Check sheet for the modelled part. Datum: model origin and axes. Units: mm. Give positions to 0.01 mm unless a question says otherwise; leave off trailing zeros. Order: outer loops, then holes, each group sorted by start corner. A loop starts at its lowest first (then second) coordinate and runs counter-clockwise, first axis right, second up.
Autodesk Inventor part; units mm, degrees
ref_plane "YZ Plane" through (0, 0, 0) normal (1, 0, 0) x (0, 1, 0)
ref_plane "XZ Plane" through (0, 0, 0) normal (0, 1, 0) x (-1, 0, 0)
ref_plane "XY Plane" through (0, 0, 0) normal (0, 0, 1) x (1, 0, 0)
sketch "main" plane through (0, 0, 0) normal (0, 0, 1) x (1, 0, 0)
  circle A0 centre (2.6045, 11.9092) radius 2.1844
  circle A1 centre (-3.5552, 26.8777) radius 2.0955
  arc A2 (-0.6729, 30.669) -> (-7.4873, 29.5648) centre (-3.5552, 26.8777) ccw
  circle A3 centre (19.8371, 7.1) radius 2.0955
  arc A4 (24.7659, 3.0962) -> (23.6801, 12.155) centre (19.8371, 7.1) ccw
  circle A5 centre (-16.2552, -5.1047) radius 2.1844
  circle A6 centre (-0.7959, -18.3) radius 2.0955
  arc A7 (-0.0936, -24.6111) -> (4.1329, -22.3038) centre (-0.7959, -18.3) ccw
  circle A8 centre (-25.6851, -13.6116) radius 2.1844
  line L0 (-34.4127, -28.4296) -> (-0.0936, -24.6111)
  circle A9 centre (-35.1149, -22.1186) radius 2.1844
  arc A10 (-40.3577, -18.5358) -> (-34.4127, -28.4296) centre (-35.1149, -22.1186) ccw
  line L1 (-7.4873, 29.5648) -> (-40.3577, -18.5358)
  line L2 (24.7659, 3.0962) -> (4.1329, -22.3038)
  line L3 (-0.6729, 30.669) -> (23.6801, 12.155)
  point P0 (-5.4325, -4.0149)
  point P1 (-6.8254, 3.4022)
  dimension "d2" = 4.191
  dimension "d3" = 12.7
  dimension "d5" = 12.7
  dimension "d6" = 12.7
  dimension "d8" = 4.191
  dimension "d9" = 9.525
  dimension "d10" = 4.191
  dimension "d13" = 4.3688
sketch "Sketch1" plane through (0, 0, 0) normal (0, 0, 1) x (1, 0, 0)
  circle A0 centre (2.6045, 11.9092) radius 2.1844
  circle A1 centre (-3.5552, 26.8777) radius 2.0955
  arc A2 (-0.6729, 30.669) -> (-7.4873, 29.5648) centre (-3.5552, 26.8777) ccw
  circle A3 centre (19.8371, 7.1) radius 2.0955
  arc A4 (24.7659, 3.0962) -> (23.6801, 12.155) centre (19.8371, 7.1) ccw
  circle A5 centre (-16.2552, -5.1047) radius 2.1844
  circle A6 centre (-0.7959, -18.3) radius 2.0955
  arc A7 (-0.0936, -24.6111) -> (4.1329, -22.3038) centre (-0.7959, -18.3) ccw
  circle A8 centre (-25.6851, -13.6116) radius 2.1844
  line L0 (-34.4127, -28.4296) -> (-0.0936, -24.6111)
  circle A9 centre (-35.1149, -22.1186) radius 2.1844
  arc A10 (-40.3577, -18.5358) -> (-34.4127, -28.4296) centre (-35.1149, -22.1186) ccw
  line L1 (-7.4873, 29.5648) -> (-40.3577, -18.5358)
  line L2 (24.7659, 3.0962) -> (4.1329, -22.3038)
  line L3 (-0.6729, 30.669) -> (23.6801, 12.155)
  point P0 (0, 0)
extrude "Extrusion1" add sketch "Sketch1" along normal blind 1.5875
properties part number "Gearbox" material "Acetal Resin, White"
(1) Release check for a two-part mould opening along Y. For faces 1 (the face through (-8, -5, 0)), 2 (the face through (-23.692, 5.851, 0.783)), 3 (the face through (-36.85, -20.79, 0.78)), 4 (the face through (-40.505, -25.476, 0.783)) record: released by +Y, released by -Y, zero draft, split by the parting line, or undercut.
Response values:
face 1: zero draft
face 2: released by +Y
face 3: undercut
face 4: split by the parting line
(2) Cross-section at C-C on x = -9.5. Enter the section's corners in (y, z), then the cut area to 3 significant figures.
Response values:
outline: (-25.66, 0) - (26.62, 0) - (26.62, 1.59) - (-25.66, 1.59) - close
area: 83.0 mm2
(3) Cross-section at D-D on y = 21.5. Enter the section's corners in (x, z).
Response values:
outline: (-13, 0) - (11.39, 0) - (11.39, 1.59) - (-13, 1.59) - close
(4) Cross-section at B-B on z = 0.9. Enter the section's corners in (x, y) (1 decimal), then the cut area to 3 significant figures.
Response values:
outline: (-40.4, -18.5) arc R6.3 ccw to (-34.4, -28.4) - (-0.1, -24.6) arc R6.4 ccw to (4.1, -22.3) - (24.8, 3.1) arc R6.3 ccw to (23.7, 12.2) - (-0.7, 30.7) arc R4.8 ccw to (-7.5, 29.6) - close; hole circle Ø4.4 at (-35.1, -22.1); hole circle Ø4.4 at (-25.7, -13.6); hole circle Ø4.4 at (-16.3, -5.1); hole circle Ø4.2 at (-3.6, 26.9); hole circle Ø4.2 at (-0.8, -18.3); hole circle Ø4.4 at (2.6, 11.9); hole circle Ø4.2 at (19.8, 7.1)
area: 2,210 mm2
(5) Cross-section at A-A on y = 13. Enter the section's corners in (x, z), then the cut area to 3 significant figures.
Response values:
outline: (-18.81, 0) - (0.71, 0) - (0.71, 1.59) - (-18.81, 1.59) - close; (4.5, 0) - (22.57, 0) - (22.57, 1.59) - (4.5, 1.59) - close
area: 59.7 mm2
(6) Material ranges on L1, parallel to Y at x = -2.5, z = 0.6; L2, parallel to X at y = 7.5, z = 1.2; L3, parallel to X at y = -17.5, z = 0.7, recorded low to high.
Response values:
L1: y = -24.88 to -19.52, -17.08 to 25.07, 28.69 to 31.52
L2: x = -22.57 to 17.78, 21.89 to 26.17
L3: x = -39.65 to -2.73, 1.14 to 8.04
